from build123d import *

# Parameters (mm, degrees)
SKETCH1_R           = 3.3
SKETCH1_R_2         = 1.25
BOSS_EXTRUDE1_DEPTH = 0.2


with BuildPart() as part:
    # Sketch1 → Boss-Extrude1 (new body)
    with BuildSketch(Plane(origin=(0, 0, 0), x_dir=(1, 0, 0), z_dir=(0, 1, 0))):
        with BuildLine():
            Line((-37.367243025, 42.925002652), (-37.367243025, -3.074997348))
            ThreePointArc((-37.367243025, -3.074997348), (-36.781456588, -4.48921091), (-35.367243025, -5.074997348))
            Line((-35.367243025, -5.074997348), (10.632756975, -5.074997348))
            ThreePointArc((10.632756975, -5.074997348), (12.046970537, -4.48921091), (12.632756975, -3.074997348))
            Line((12.632756975, -3.074997348), (12.632756975, 42.925002652))
            ThreePointArc((12.632756975, 42.925002652), (12.046970537, 44.339216214), (10.632756975, 44.925002652))
            Line((10.632756975, 44.925002652), (-35.367243025, 44.925002652))
            ThreePointArc((-35.367243025, 44.925002652), (-36.781456588, 44.339216214), (-37.367243025, 42.925002652))
        make_face()
        with Locations(Location((-17.667243025, 25.225002652, 0), (0, 0, 270))):
            Circle(SKETCH1_R, mode=Mode.SUBTRACT)
        with Locations(Location((7.332756975, 16.987502652, 0), (0, 0, 270))):
            Circle(SKETCH1_R_2, mode=Mode.SUBTRACT)
        with Locations(Location((7.332756975, 28.162502652, 0), (0, 0, 270))):
            Circle(SKETCH1_R_2, mode=Mode.SUBTRACT)
        with Locations(Location((7.332756975, 39.337502652, 0), (0, 0, 270))):
            Circle(SKETCH1_R_2, mode=Mode.SUBTRACT)
        with Locations(Location((7.332756975, 5.812502652, 0), (0, 0, 270))):
            Circle(SKETCH1_R_2, mode=Mode.SUBTRACT)
        with Locations(Location((1.745256975, 0.225002652, 0), (0, 0, 270))):
            Circle(SKETCH1_R_2, mode=Mode.SUBTRACT)
        with Locations(Location((-9.429743025, 0.225002652, 0), (0, 0, 270))):
            Circle(SKETCH1_R_2, mode=Mode.SUBTRACT)
        with Locations(Location((-20.604743025, 0.225002652, 0), (0, 0, 270))):
            Circle(SKETCH1_R_2, mode=Mode.SUBTRACT)
        with Locations(Location((-31.779743025, 0.225002652, 0), (0, 0, 270))):
            Circle(SKETCH1_R_2, mode=Mode.SUBTRACT)
    extrude(amount=BOSS_EXTRUDE1_DEPTH)


solid = part.part
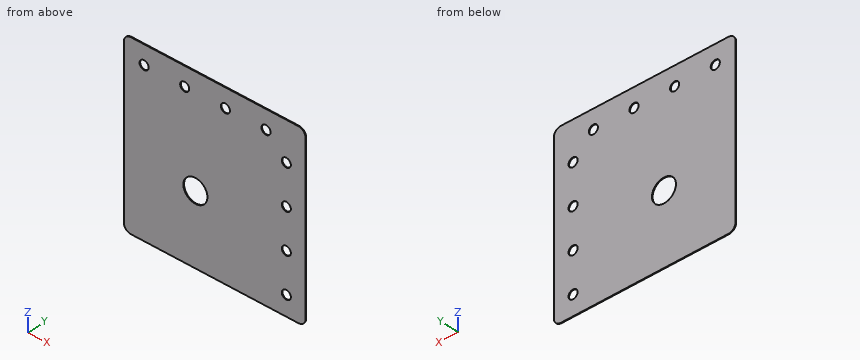
For this review, take the finished solid that the model builds, in its own axes (mm). Round coordinates to 2 decimals unless told otherwise and drop trailing zeros. Loops run counter-clockwise (first coordinate to the right, second up) from the corner with the lowest first, then second, coordinate; pieces in that order, holes last. Notation, with made-up numbers: (-40, 0.25) - (-23, 0.25) arc R20 cw to (-23, 5.25) - close; hole circle Ø7 at (22, -39). An arc over 180 degrees is marked (long way). One line per item, written item: value. Start each with the question number.
Item 1: Take a section at B-B (z = -23). Give the boundary of the cut face in (x, y), plus the area to 3 significant figures.
Item 2: For L1, parallel to X at y = 0.15, z = -24; L2, parallel to Z at x = -32, y = 0.1 (3 decimals); L3, parallel to X at y = 0.1, z = -39, list the stretches that pass through material, from the lowest coordinate up.
Item 3: Take a section at C-C (y = 0.15). State how many separate pieces and enclosed holes the cut face has, plus the area to 3 significant figures.
Item 4: Take a section at A-A (x = -15). Give the boundary of the cut face in (y, z) (3 decimals).
Answer below:
1. outline: (-37.37, 0) - (-20.1, 0) - (-20.1, 0.2) - (-37.37, 0.2) - close; (-15.23, 0) - (12.63, 0) - (12.63, 0.2) - (-15.23, 0.2) - close
1. area: 9.03 mm2
2. L1: x = -37.37 to -20.73, -14.6 to 12.63
2. L2: z = -44.925 to -1.455, 1.005 to 5.075
2. L3: x = -37.37 to 6.13, 8.54 to 12.63
3. separate pieces: 1
3. enclosed holes: 9
3. area: 2,420 mm2
4. outline: (0, -44.925) - (0.2, -44.925) - (0.2, -27.168) - (0, -27.168) - close; (0, -23.282) - (0.2, -23.282) - (0.2, 5.075) - (0, 5.075) - close
